Could you check a few things on this model? Use its own coordinates, in mm. Round coordinates to 2 decimals unless told otherwise and drop trailing zeros. Order: outer loops, then holes, each group sorted by start corner. A loop starts at its lowest first (then second) coordinate and runs counter-clockwise, first axis right, second up.
```python
from build123d import *

# Parameters (mm, degrees)
SKETCH_1_R                   = 100
EXTRUDE_1_DEPTH              = 5
HOLE_WIZARD_M3_1_D           = 2.5
HOLE_WIZARD_M3_1_CSINK_D     = 3.05
HOLE_WIZARD_M3_1_CSINK_ANGLE = 90
SKETCH_5_R                   = 12.5
CUT_EXTRUDE_1_DEPTH          = 142.509716981
HOLE_WIZARD_M4_2_D           = 3.3
HOLE_WIZARD_M4_2_DEPTH       = 5
HOLE_WIZARD_M4_2_CSINK_D     = 4.05
HOLE_WIZARD_M4_2_CSINK_ANGLE = 90


# Read off the part's stored shape, not the designer's step: M3 螺纹孔2
with BuildPart() as part:
    # 草图1 → 凸台-拉伸1 (new body)
    with BuildSketch(Plane(origin=(0, 0, 0), x_dir=(1, 0, 0), z_dir=(0, 1, 0))):
        with Locations(Location((0, 0, 0), (0, 0, 270))):
            Circle(SKETCH_1_R)
    extrude(amount=EXTRUDE_1_DEPTH)

    # M3 螺纹孔1 (through all)
    with Locations(Plane(origin=(0, 5, 0), x_dir=(1, 0, 0), z_dir=(0, 1, 0))):
        with Locations((0, 20), (17.320508076, -10), (-17.320508076, -10)):
            CounterSinkHole(HOLE_WIZARD_M3_1_D / 2, HOLE_WIZARD_M3_1_CSINK_D / 2, counter_sink_angle=HOLE_WIZARD_M3_1_CSINK_ANGLE)

    # 草图5 → 切除-拉伸1 (cut, through all)
    with BuildSketch(Plane(origin=(0, 5, 0), x_dir=(1, 0, 0), z_dir=(0, 1, 0))):
        with Locations(Location((0, 0, 0), (0, 0, 270))):
            Circle(SKETCH_5_R)
    extrude(amount=-CUT_EXTRUDE_1_DEPTH, mode=Mode.SUBTRACT)

    # M4 螺纹孔2
    with Locations(Plane(origin=(0, 5, 0), x_dir=(1, 0, 0), z_dir=(0, 1, 0))):
        with Locations((0, 0), (-28.35, 85), (28.35, 85), (28.35, -85), (-28.35, -85), (-28.35, 59), (28.35, 59), (-28.35, -59), (28.35, -59)):
            CounterSinkHole(HOLE_WIZARD_M4_2_D / 2, HOLE_WIZARD_M4_2_CSINK_D / 2, depth=HOLE_WIZARD_M4_2_DEPTH, counter_sink_angle=HOLE_WIZARD_M4_2_CSINK_ANGLE)

    # M3 螺纹孔2 outline → M3 螺纹孔2 (revolve, cut)
    with BuildSketch(Plane(origin=(4, 0, 58), x_dir=(1, 0, 0), z_dir=(0, 0, 1))):
        Polygon((0, 0), (1.25, 0), (1.25, 4.725), (1.525, 5), (0, 5), align=None)
    revolve(axis=Axis((4, 0, 58), (0, 1, 0)), mode=Mode.SUBTRACT)

    # Hole Wizard M3 _2 2 outline → Hole Wizard M3 _2 2 (revolve, cut)
    with BuildSketch(Plane(origin=(-4, 0, 58), x_dir=(1, 0, 0), z_dir=(0, 0, 1))):
        Polygon((0, 0), (1.25, 0), (1.25, 4.725), (1.525, 5), (0, 5), align=None)
    revolve(axis=Axis((-4, 0, 58), (0, 1, 0)), mode=Mode.SUBTRACT)

    # Hole Wizard M3 _2 3 outline → Hole Wizard M3 _2 3 (revolve, cut)
    with BuildSketch(Plane(origin=(4, 0, -58), x_dir=(1, 0, 0), z_dir=(0, 0, 1))):
        Polygon((0, 0), (1.25, 0), (1.25, 4.725), (1.525, 5), (0, 5), align=None)
    revolve(axis=Axis((4, 0, -58), (0, 1, 0)), mode=Mode.SUBTRACT)

    # Hole Wizard M3 _2 4 outline → Hole Wizard M3 _2 4 (revolve, cut)
    with BuildSketch(Plane(origin=(-4, 0, -58), x_dir=(1, 0, 0), z_dir=(0, 0, 1))):
        Polygon((0, 0), (1.25, 0), (1.25, 4.725), (1.525, 5), (0, 5), align=None)
    revolve(axis=Axis((-4, 0, -58), (0, 1, 0)), mode=Mode.SUBTRACT)


solid = part.part
```
Q1. I need wall thicknesses on L1, parallel to X at y = 3, z = 0; L2, parallel to X at y = 1.85, z = 85; L3, parallel to X at y = 3.3, z = 59. Which ranges of each line are inside material? Lowest first, please.
Q2. We'd pull the mould along X, two halves only. Please class faces 1 (the cylindrical face through (3.755, 2.535, 11.923)), 2 (the flat face through (-21, 5, -1)), 3 (the cylindrical face through (30.04, 2.46, 95.38)): released by +X, released by -X, zero draft, split by the parting line, or undercut.
Q3. Imagine slicing it at A-A, the plane y = 1.2. State how many separate pieces and enclosed holes the cut face has, then the cut area to 3 significant figures.
Q4. For P1, Ø1, axis at x = -11, y = 3.5, coming from the +Z side; P2, Ø2.5, axis at x = -28.35, z = 85, coming from the -Y side; P3, Ø1.5, axis at x = -56.5, y = 3, coming from the -Z side; P4, Ø12, axis at x = 3.5, z = 74, coming from the -Y side, each with a flat end and sliding along its axis, tell me the tip position at first contact or that it passes through.
Q5. Imagine slicing it at C-C, the plane x = -80.5. Please give me the cut outline in (y, z).
Q6. Imagine slicing it at D-D, the plane z = 27.5. Please give me the cut outline in (x, y).
Q7. Imagine slicing it at B-B, the plane z = -1.5. Please give me the cut outline in (x, y), then the cut area to 3 significant figures.
Filled in:
1. L1: x = -100 to -12.5, 12.5 to 100
1. L2: x = -52.68 to -30, -26.7 to 26.7, 30 to 52.68
1. L3: x = -80.74 to -30, -26.7 to -4.75, -3.25 to 3.25, 4.75 to 26.7, 30 to 80.74
2. face 1: undercut
2. face 2: zero draft
2. face 3: split by the parting line
3. separate pieces: 1
3. enclosed holes: 16
3. area: 30,800 mm2
4. P1: stops at z = 99.45
4. P2: passes through
4. P3: stops at z = -83.02
4. P4: stops at y = 0
5. outline: (0, -59.33) - (5, -59.33) - (5, 59.33) - (0, 59.33) - close
6. outline: (-96.14, 0) - (96.14, 0) - (96.14, 5) - (-96.14, 5) - close
7. outline: (-99.99, 0) - (-12.41, 0) - (-12.41, 5) - (-99.99, 5) - close; (12.41, 0) - (99.99, 0) - (99.99, 5) - (12.41, 5) - close
7. area: 876 mm2
